from build123d import *

# Parameters (mm, degrees)
ESBO_O1_R             = 75
ESBO_O1_R_2           = 15
EXTRUS_O1_DEPTH       = 6
ESBO_O2_R             = 5.25
CORTE_EXTRUS_O1_DEPTH = 107.742681248
CIRPATTERN1_COUNT     = 3
ESBO_O3_R             = 94.650975841
ESBO_O3_R_2           = 75
CORTE_EXTRUS_O3_DEPTH = 107.742681248


with BuildPart() as part:
    # Esboço1 → Extrusão1 (new, symmetric)
    with BuildSketch(Plane.XY):
        Circle(ESBO_O1_R)
        Circle(ESBO_O1_R_2, mode=Mode.SUBTRACT)
    extrude(amount=EXTRUS_O1_DEPTH, both=True)

    # Esboço2 → Corte-extrusão1 (cut, through all)
    with BuildSketch(Plane.XY.offset(6)):
        with Locations((0, 65)):
            Circle(ESBO_O2_R)
    corte_extrus_o1 = extrude(amount=-CORTE_EXTRUS_O1_DEPTH, mode=Mode.SUBTRACT)

    # CirPattern1: Corte-extrusão1 ×3 about axis
    cirpattern1_axis = Axis((0, 0, 0), (0, 0, 1))
    for i in range(1, CIRPATTERN1_COUNT):
        add(corte_extrus_o1.rotate(cirpattern1_axis, i * 360 / CIRPATTERN1_COUNT), mode=Mode.SUBTRACT)

    # Esboço3 → Corte-extrusão3 (cut, through all)
    # profile 1 of 4: a face of its own
    with BuildSketch(Plane.XY.offset(6)):
        Circle(ESBO_O3_R)
        Circle(ESBO_O3_R_2, mode=Mode.SUBTRACT)
    # profile 2 of 4: a face of its own
    with BuildSketch(Plane.XY.offset(6)):
        with BuildLine():
            ThreePointArc((-11.389775772, 68.231933262), (-9.651857518, 71.856677855), (-6.801268948, 74.690981656))
            ThreePointArc((-6.801268948, 74.690981656), (-64.951905284, 37.5), (-68.084922021, -31.455419141))
            ThreePointArc((-68.084922021, -31.455419141), (-67.055637213, -27.569585123), (-64.78547544, -24.252131468))
            Line((-64.78547544, -24.252131468), (-55.572211308, -14.764123082))
            ThreePointArc((-55.572211308, -14.764123082), (-49.796460718, 28.75), (-15, 55.509008278))
            Line((-15, 55.509008278), (-11.389775772, 68.231933262))
        make_face()
    # profile 3 of 4: a face of its own
    with BuildSketch(Plane.XY.offset(6)):
        with BuildLine():
            ThreePointArc((-53.395699668, -43.979801793), (-57.403779695, -44.287092732), (-61.283653073, -43.235562515))
            ThreePointArc((-61.283653073, -43.235562515), (0, -75), (61.283653073, -43.235562515))
            ThreePointArc((61.283653073, -43.235562515), (57.403779695, -44.287092732), (53.395699668, -43.979801793))
            Line((53.395699668, -43.979801793), (40.572211308, -40.744885196))
            ThreePointArc((40.572211308, -40.744885196), (0, -57.5), (-40.572211308, -40.744885196))
            Line((-40.572211308, -40.744885196), (-53.395699668, -43.979801793))
        make_face()
    # profile 4 of 4: a face of its own
    with BuildSketch(Plane.XY.offset(6)):
        with BuildLine():
            ThreePointArc((6.801268948, 74.690981656), (9.651857518, 71.856677855), (11.389775772, 68.231933262))
            Line((11.389775772, 68.231933262), (15, 55.509008278))
            ThreePointArc((15, 55.509008278), (45.654955919, 34.955328635), (57.5, 0))
            ThreePointArc((57.5, 0), (57.016015952, -7.444724636), (55.572211308, -14.764123082))
            Line((55.572211308, -14.764123082), (64.78547544, -24.252131468))
            ThreePointArc((64.78547544, -24.252131468), (67.055637213, -27.569585123), (68.084922021, -31.455419141))
            ThreePointArc((68.084922021, -31.455419141), (73.250833277, -16.10327371), (75, 0))
            ThreePointArc((75, 0), (55.385445611, 50.571260756), (6.801268948, 74.690981656))
        make_face()
    extrude(amount=-CORTE_EXTRUS_O3_DEPTH, mode=Mode.SUBTRACT)


solid = part.part
Check sheet for the modelled part. Datum: model origin and axes. Units: mm. A direction names the side the tool comes from. Coordinates: 2 decimals unless noted, no trailing zeros. Loops run counter-clockwise (first coordinate to the right, second up) from the corner with the lowest first, then second, coordinate; pieces in that order, holes last. Notation, with made-up numbers: (47, 2) -> (66, 2) arc R21 ccw to (66, 9) -> close; hole circle Ø2 at (35.5, -30.5). An arc over 180 degrees is marked (long way). Answer in a Markdown table with one row per item.
1. Release check for a two-part mould opening along X. For faces 6 (the face through (0, 75, 0)), 7 (the face through (61.3, -30.92, 0.08)), 8 (the face through (-67.08, -27.62, 0.08)) record: released by +X, released by -X, zero draft, split by the parting line, or undercut.
Check values:
| item | result |
|---|---|
| face 6 | split by the parting line |
| face 7 | undercut |
| face 8 | released by -X |
2. Access from +Z, -Z, +X, -X, +Y, -Y to the whole of each face (thin tool, end or side, straight path). Record for faces 1 (the face through (-16, -5, -6)), 2 (the face through (-60.24, -19.57, 0.08)), 3 (the face through (-46.89, -42.34, 0.08)), 4 (the face through (60.11, -19.44, 0.08)), 5 (the face through (9.62, 71.9, 0.08)).
Check values:
| item | result |
|---|---|
| face 1 | -Z, +X, -X, +Y, -Y |
| face 2 | +Z, -Z, -X |
| face 3 | +Z, -Z, -Y |
| face 4 | +Z, -Z, +X |
| face 5 | +Z, -Z, +X, +Y |
3. Material ranges on line 1 along Y through (x, z) = (2.5, 4.25); line 2 along Y through (x, z) = (0, 1.5); line 3 along Y through (x, z) = (-60.5, -3.5), recorded low to high. Write a range as [from, to].
Check values:
| item | result |
|---|---|
| line 1 | y = [-57.45, -14.79], [14.79, 60.38], [69.62, 74.96] |
| line 2 | y = [-57.5, -15], [15, 59.75], [70.25, 75] |
| line 3 | y = [-43.57, -35.64], [-29.36, -19.84] |
4. Sectioned sample at A-A, the plane x = 0. Record the boundary of the cut face in (y, z).
Check values:
| item | result |
|---|---|
| outline | (-57.5, -6) -> (-15, -6) -> (-15, 6) -> (-57.5, 6) -> close; (15, -6) -> (59.75, -6) -> (59.75, 6) -> (15, 6) -> close; (70.25, -6) -> (75, -6) -> (75, 6) -> (70.25, 6) -> close |
5. Sectioned sample at D-D, the plane y = -48. Record the boundary of the cut face in (x, z), then the cut area to 3 significant figures.
Check values:
| item | result |
|---|---|
| outline | (-31.66, -6) -> (31.66, -6) -> (31.66, 6) -> (-31.66, 6) -> close |
| area | 760 mm2 |
6. Go/stop test with flat-tipped pins: pin 1 (2 mm diameter, centred on x = -14.5, z = 1, fed in from -Y); pin 2 (4 mm diameter, centred on y = 21, z = -2, fed in from -X); pin 3 (3 mm diameter, centred on x = 30, z = 4, fed in from -Y). Record where each tip stops, or that it passes through.
Check values:
| item | result |
|---|---|
| pin 1 | stops at y = -55.89 |
| pin 2 | stops at x = -54.27 |
| pin 3 | stops at y = -49.94 |
7. Sectioned sample at C-C, the plane z = 1.75. Record the boundary of the cut face in (x, y).
Check values:
| item | result |
|---|---|
| outline | (-68.08, -31.46) arc R75 ccw to (-61.28, -43.24) arc R11.84 ccw to (-53.4, -43.98) -> (-40.57, -40.74) arc R57.5 ccw to (40.57, -40.74) -> (53.4, -43.98) arc R11.84 ccw to (61.28, -43.24) arc R75 ccw to (68.08, -31.46) arc R11.84 ccw to (64.79, -24.25) -> (55.57, -14.76) arc R57.5 ccw to (15, 55.51) -> (11.39, 68.23) arc R11.84 ccw to (6.8, 74.69) arc R75 ccw to (-6.8, 74.69) arc R11.84 ccw to (-11.39, 68.23) -> (-15, 55.51) arc R57.5 ccw to (-55.57, -14.76) -> (-64.79, -24.25) arc R11.84 ccw to start; hole circle Ø10.5 at (-56.29, -32.5); hole circle Ø30 at (0, 0); hole circle Ø10.5 at (0, 65); hole circle Ø10.5 at (56.29, -32.5) |
8. Sectioned sample at B-B, the plane y = 65. Record the boundary of the cut face in (x, z), then the cut area to 3 significant figures.
Check values:
| item | result |
|---|---|
| outline | (-12.31, -6) -> (-5.25, -6) -> (-5.25, 6) -> (-12.31, 6) -> close; (5.25, -6) -> (12.31, -6) -> (12.31, 6) -> (5.25, 6) -> close |
| area | 169 mm2 |
